```python
from build123d import *

# Parameters (mm, degrees)
SKETCH2_R           = 6.35
BOSS_EXTRUDE1_DEPTH = 6.35
SKETCH3_W           = 101.6
SKETCH3_H           = 76.2
BOSS_EXTRUDE3_DEPTH = 47.8
CUT_EXTRUDE1_DEPTH  = 449.400286045


with BuildPart() as part:
    # Sketch2 → Boss-Extrude1 (new body)
    with BuildSketch(Plane.XY):
        Polygon((-50.8, 0), (50.8, 0), (50.8, 161.115902063), (194.484097937, 17.431804126), (266.326146906, 89.273853094), (50.8, 304.8), (-50.8, 304.8), (-266.326146906, 89.273853094), (-194.484097937, 17.431804126), (-50.8, 161.115902063), align=None)
        with Locations((212.444610179, 107.234365336)):
            Circle(SKETCH2_R, mode=Mode.SUBTRACT)
        with Locations((172.033457634, 147.645517881)):
            Circle(SKETCH2_R, mode=Mode.SUBTRACT)
        with Locations((131.62230509, 188.056670426)):
            Circle(SKETCH2_R, mode=Mode.SUBTRACT)
        with Locations(Location((136.11243315, 111.724493397, 0), (0, 0, 180))):
            Circle(SKETCH2_R, mode=Mode.SUBTRACT)
        with Locations(Location((95.701280605, 152.135645942, 0), (0, 0, 180))):
            Circle(SKETCH2_R, mode=Mode.SUBTRACT)
        with Locations(Location((176.523585695, 71.313340852, 0), (0, 0, 180))):
            Circle(SKETCH2_R, mode=Mode.SUBTRACT)
        with Locations((25.4, 50.8)):
            Circle(SKETCH2_R, mode=Mode.SUBTRACT)
        with Locations((25.4, 152.4)):
            Circle(SKETCH2_R, mode=Mode.SUBTRACT)
        with Locations((25.4, 254)):
            Circle(SKETCH2_R, mode=Mode.SUBTRACT)
        with Locations(Location((-25.4, 254, 0), (0, 0, 180))):
            Circle(SKETCH2_R, mode=Mode.SUBTRACT)
        with Locations(Location((-25.4, 152.4, 0), (0, 0, 180))):
            Circle(SKETCH2_R, mode=Mode.SUBTRACT)
        with Locations(Location((-25.4, 50.8, 0), (0, 0, 180))):
            Circle(SKETCH2_R, mode=Mode.SUBTRACT)
        with Locations((-176.523585695, 71.313340852)):
            Circle(SKETCH2_R, mode=Mode.SUBTRACT)
        with Locations((-95.701280605, 152.135645942)):
            Circle(SKETCH2_R, mode=Mode.SUBTRACT)
        with Locations((-136.11243315, 111.724493397)):
            Circle(SKETCH2_R, mode=Mode.SUBTRACT)
        with Locations(Location((-131.62230509, 188.056670426, 0), (0, 0, 180))):
            Circle(SKETCH2_R, mode=Mode.SUBTRACT)
        with Locations(Location((-172.033457634, 147.645517881, 0), (0, 0, 180))):
            Circle(SKETCH2_R, mode=Mode.SUBTRACT)
        with Locations(Location((-212.444610179, 107.234365336, 0), (0, 0, 180))):
            Circle(SKETCH2_R, mode=Mode.SUBTRACT)
    extrude(amount=BOSS_EXTRUDE1_DEPTH)

    # Sketch3 → Boss-Extrude3 (add)
    with BuildSketch(Plane(origin=(0, 304.8, 0), x_dir=(1, 0, 0), z_dir=(0, 1, 0))):
        with Locations((0, -38.1)):
            Rectangle(SKETCH3_W, SKETCH3_H)
    extrude(amount=BOSS_EXTRUDE3_DEPTH)

    # Sketch4 → Cut-Extrude1 (cut, through all)
    with BuildSketch(Plane.XY.offset(76.2)):
        with BuildLine():
            Line((-31.068100257, 352.6), (31.068100257, 352.6))
            ThreePointArc((31.068100257, 352.6), (0, 314.305105316), (-31.068100257, 352.6))
        make_face()
    extrude(amount=-CUT_EXTRUDE1_DEPTH, mode=Mode.SUBTRACT)


solid = part.part
```
Input: part model. Units: mm. Frame: model coordinates. A direction names the side the tool comes from. Coordinates: 2 decimals unless noted, no trailing zeros. Order: outer loops, then holes, each group sorted by start corner. A loop starts at its lowest first (then second) coordinate and runs counter-clockwise, first axis right, second up. Notation, with made-up numbers: (3, 89) - (9, 89) arc R25 cw to (9, 103) - close; hole circle Ø2 at (-22.75, 35). An arc over 180 degrees is marked (long way). Put each result on its own line as item: value.
1. Cut plane C-C on y = 50.8. Return the cut outline in (x, z).
Report:
outline: (-227.85, 0) - (-161.12, 0) - (-161.12, 6.35) - (-227.85, 6.35) - close; (-50.8, 0) - (-31.75, 0) - (-31.75, 6.35) - (-50.8, 6.35) - close; (-19.05, 0) - (19.05, 0) - (19.05, 6.35) - (-19.05, 6.35) - close; (31.75, 0) - (50.8, 0) - (50.8, 6.35) - (31.75, 6.35) - close; (161.12, 0) - (227.85, 0) - (227.85, 6.35) - (161.12, 6.35) - close
2. Cut plane B-B on y = 128.5. Return the cut outline in (x, z).
Report:
outline: (-227.1, 0) - (-83.42, 0) - (-83.42, 6.35) - (-227.1, 6.35) - close; (-50.8, 0) - (50.8, 0) - (50.8, 6.35) - (-50.8, 6.35) - close; (83.42, 0) - (227.1, 0) - (227.1, 6.35) - (83.42, 6.35) - close
3. Draft query along Y for faces 3 (the face through (-24.6, 247.7, 3.1)), 4 (the face through (-4, 155, 6.35)), 5 (the face through (121.636, 90.28, 3.131)). Return one class per face: pulls with the +Y half, pulls with the -Y half, needs draft (parallel to the pull), parting line crosses it, or undercut.
Report:
face 3: undercut
face 4: needs draft
face 5: pulls with the -Y half
4. Cut plane A-A on x = 25.4. Return the cut outline in (y, z).
Report:
outline: (0, 0) - (44.45, 0) - (44.45, 6.35) - (0, 6.35) - close; (57.15, 0) - (146.05, 0) - (146.05, 6.35) - (57.15, 6.35) - close; (158.75, 0) - (247.65, 0) - (247.65, 6.35) - (158.75, 6.35) - close; (260.35, 0) - (327.01, 0) - (327.01, 76.2) - (304.8, 76.2) - (304.8, 6.35) - (260.35, 6.35) - close
5. Reachability of faces 1 (the face through (-123.648, 88.268, 3.131)), 2 (the face through (20.72, 156.69, 3.13)) from +Z, -Z, +X, -X, +Y, -Y: full face, straight path, thin tool, end or side. Return the list, or none.
Report:
face 1: +Z, -Z, -Y
face 2: +Z, -Z
6. Line query: line 1 along Z through (x, y) = (-144, 188.5); line 2 along X through (y, z) = (81.5, 6); line 3 along Y through (x, z) = (-1, 63). Output: solid intervals per line, ascending.
Report:
line 1: z = 0 to 6.35
line 2: x = -258.55 to -130.42, -50.8 to 50.8, 130.42 to 258.55
line 3: y = 304.8 to 314.32
7. Cut plane D-D on z = 54. Return the cut outline in (x, y).
Report:
outline: (-50.8, 304.8) - (50.8, 304.8) - (50.8, 352.6) - (31.07, 352.6) arc R31.75 cw (long way) to (-31.07, 352.6) - (-50.8, 352.6) - close
8. Contact query for flat-ended pins moving along their axis: pin 1 Ø1 at (x, y) = (103.5, 252) entering from +Z; pin 2 Ø10 at (x, y) = (-25.4, 254) entering from +Z; pin 3 Ø14.5 at (x, y) = (-136.11, 111.72) entering from -Z; pin 4 Ø3 at (y, z) = (68.5, 3.5) entering from -X. Output: stop coordinate, or through.
Report:
pin 1: stops at z = 6.35
pin 2: passes through
pin 3: stops at z = 0
pin 4: stops at x = -247.05
